```python
from build123d import *

# Parameters (mm, degrees)
F0_R     = 190.5
F0_R_2   = 165.1
F1_DEPTH = 254
F2_R     = 6.096
F3_DEPTH = 12.7


with BuildPart() as f1:
    # F0 (on Top) → F1 (new body)
    with BuildSketch(Plane.XY):
        Circle(F0_R)
        Circle(F0_R_2, mode=Mode.SUBTRACT)
    extrude(amount=-F1_DEPTH)

    # F2 (on Top) → F3 (cut)
    with BuildSketch(Plane.XY):
        with Locations((0, 178.42484)):
            Circle(F2_R)
        with Locations((-89.21242, 154.5204441062)):
            Circle(F2_R)
        with Locations((-154.5204441062, 89.21242)):
            Circle(F2_R)
        with Locations((-178.42484, 0)):
            Circle(F2_R)
        with Locations((-154.5204441062, -89.21242)):
            Circle(F2_R)
        with Locations((-89.21242, -154.5204441062)):
            Circle(F2_R)
        with Locations((0, -178.42484)):
            Circle(F2_R)
        with Locations((89.21242, -154.5204441062)):
            Circle(F2_R)
        with Locations((154.5204441062, -89.21242)):
            Circle(F2_R)
        with Locations((178.42484, 0)):
            Circle(F2_R)
        with Locations((154.5204441062, 89.21242)):
            Circle(F2_R)
        with Locations((89.21242, 154.5204441062)):
            Circle(F2_R)
    extrude(amount=-F3_DEPTH, mode=Mode.SUBTRACT)


solid = f1.part
```
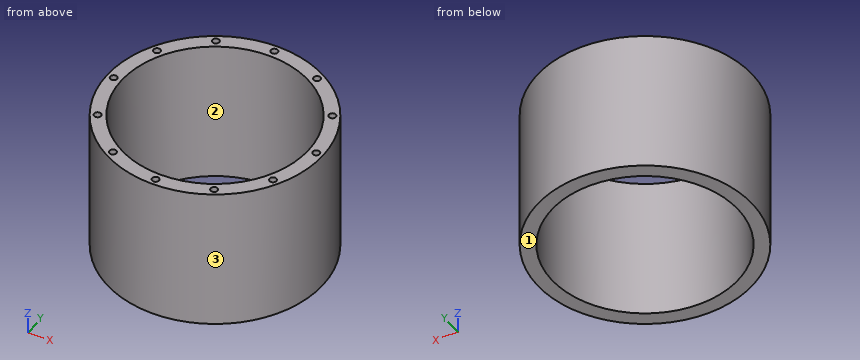
For this review, take the finished solid that the model builds, in its own axes (mm). Face numbers are marked on the shaded views. Round coordinates to 2 decimals unless told otherwise and drop trailing zeros. Loops run counter-clockwise (first coordinate to the right, second up) from the corner with the lowest first, then second, coordinate; pieces in that order, holes last.
Q1. To check wall thickness, follow line 1 along Y through (x, z) = (0, -113); line 2 along X through (y, z) = (-71.5, -232.5). State the ranges of each line that lie inside material, in increasing order.
Result sheet:
line 1: y = -190.5 to -165.1, 165.1 to 190.5
line 2: x = -176.57 to -148.81, 148.81 to 176.57
Q2. Add section C-C on z = -91. Write out the cut boundary in (x, y).
Result sheet:
outline: circle Ø381 at (0, 0); hole circle Ø330.2 at (0, 0)
Q3. Add section D-D on y = 48.5. Write out the cut boundary in (x, z).
Result sheet:
outline: (-184.22, -254) - (-157.82, -254) - (-157.82, 0) - (-184.22, 0) - close; (157.82, -254) - (184.22, -254) - (184.22, 0) - (157.82, 0) - close
Q4. Insertion check: pin 1 Ø7.5 at (x, y) = (-89.21, -154.52) entering from +Z; pin 2 Ø5 at (y, z) = (-30.5, -121) entering from -X; pin 3 Ø12 at (y, z) = (-41, -166) entering from +X. Each pin has a flat end and moves straight along its axis. Give the tip position at first contact, or say it passes through.
Result sheet:
pin 1: stops at z = -12.7
pin 2: stops at x = -188.43
pin 3: stops at x = 187.26
Q5. Mouldability with a two-part tool opening along Y and no side actions: class the marked faces 1, 2 and 3 as +Y half, -Y half, draft (parallel to the pull), parting line (faces both ways), or undercut.
Result sheet:
face 1: draft
face 2: undercut
face 3: parting line
Q6. Add section A-A on y = 0. Write out the cut boundary in (x, z).
Result sheet:
outline: (-190.5, -254) - (-165.1, -254) - (-165.1, 0) - (-172.33, 0) - (-172.33, -12.7) - (-184.52, -12.7) - (-184.52, 0) - (-190.5, 0) - close; (165.1, -254) - (190.5, -254) - (190.5, 0) - (184.52, 0) - (184.52, -12.7) - (172.33, -12.7) - (172.33, 0) - (165.1, 0) - close
